from build123d import *

# Parameters (mm, degrees)
SKETCH1_R           = 6.25
BOSS_EXTRUDE1_DEPTH = 3
BOSS_EXTRUDE2_DEPTH = 5
FILLET1_R           = 1.5


with BuildPart() as part:
    # Sketch1 → Boss-Extrude1 (new body)
    with BuildSketch(Plane(origin=(0, 0, 0), x_dir=(1, 0, 0), z_dir=(0, 1, 0))):
        with Locations(Location((0, 0, 0), (0, 0, 270))):
            Circle(SKETCH1_R)
    extrude(amount=BOSS_EXTRUDE1_DEPTH)

    # Sketch2 → Boss-Extrude2 (add)
    with BuildSketch(Plane(origin=(0, 3, 0), x_dir=(1, 0, 0), z_dir=(0, 1, 0))):
        with BuildLine():
            Line((-2, 1.5), (2, 1.5))
            ThreePointArc((2, 1.5), (0, -2.5), (-2, 1.5))
        make_face()
    extrude(amount=BOSS_EXTRUDE2_DEPTH)

    # Fillet1
    fillet1_edges = [part.edges().sort_by_distance(p)[0] for p in [
        (0, 3, -6.25),
    ]]
    fillet(fillet1_edges, radius=FILLET1_R)


solid = part.part
Source: CAD feature listing. Evaluate the final solid. Frame: model axes, mm. A direction names the side the tool comes from. Give positions to 0.01 mm unless a question says otherwise; leave off trailing zeros. Write each loop counter-clockwise with the first axis right and the second up, starting at its lowest first coordinate (ties: lowest second). Pieces come first, ordered by that corner, then holes. Notation, with made-up numbers: (-17, 57) -> (2, 57) arc R28 cw to (2, 76) -> close; hole circle Ø2 at (72, 7.25). An arc over 180 degrees is marked (long way). Return JSON: item names as keys, results as strings. Group by question number.
1. Section D-D, the plane y = 6.25. Output: boundary loops of the cut face in (x, z), then the cut area to 3 significant figures.
2. Section A-A, the plane x = 0. Output: boundary loops of the cut face in (y, z), then the cut area to 3 significant figures.
3. Material intervals for line 1 (Y direction, x = -4, z = -1.75); line 2 (X direction, y = 5.5, z = 1.5); line 3 (Z direction, x = 1.25, y = 7.25), sorted ascending. Write a range as from..to.
4. Section C-C, the plane y = 0.5. Output: boundary loops of the cut face in (x, z).
5. Access query for faces 1 (the face through (1.88, 0.74, 5.96)), 2 (the face through (0, 5, -1.5)), 3 (the face through (0, 3, -2)). Directions: +Z, -Z, +X, -X, +Y, -Y. A direction counts if a zero-diameter tool reaches every point of the face in a straight line with its end or side. Return the directions, or none.
6. Section B-B, the plane z = 0. Output: boundary loops of the cut face in (x, y), then the cut area to 3 significant figures.
7. Pin query (flat end, axial travel): pin 1 Ø1.5 at (y, z) = (3.5, -2.5) entering from -X; pin 2 Ø2 at (x, y) = (0.5, 6.5) entering from -Z. Return the tip coordinate at first contact, or that it passes through.
Determined:
{
 "1": {"outline": "(-2, -1.5) -> (2, -1.5) arc R2.5 ccw (long way) to start", "area": "16.8 mm2"},
 "2": {"outline": "(0, -6.25) -> (1.5, -6.25) arc R1.5 ccw to (3, -4.75) -> (3, -1.5) -> (8, -1.5) -> (8, 2.5) -> (3, 2.5) -> (3, 4.75) arc R1.5 ccw to (1.5, 6.25) -> (0, 6.25) -> close", "area": "56.5 mm2"},
 "3": {"line 1": "y = 0..3", "line 2": "x = -2..2", "line 3": "z = -1.5..2.17"},
 "4": {"outline": "circle Ø12.5 at (0, 0)"},
 "5": {"face 1": "+Y, -Y", "face 2": "-Z, +X, -X, +Y", "face 3": "+Y"},
 "6": {"outline": "(-6.25, 0) -> (6.25, 0) -> (6.25, 1.5) arc R1.5 ccw to (4.75, 3) -> (2.5, 3) -> (2.5, 8) -> (-2.5, 8) -> (-2.5, 3) -> (-4.75, 3) arc R1.5 ccw to (-6.25, 1.5) -> close", "area": "61.5 mm2"},
 "7": {"pin 1": "stops at x = -5.04", "pin 2": "stops at z = -1.5"}
}
